from build123d import *

# Parameters (mm, degrees)
BOSS_EXTRUDE1_DEPTH = 5
CAVITY1_START       = -0.5
CAVITY1_OUTLINE_W   = 15
CAVITY1_OUTLINE_H   = 5
CAVITY1_DEPTH       = 5


# Read off the part's stored shape, not the designer's step: Cavity1
with BuildPart() as part:
    # Sketch1 → Boss-Extrude1 (new body)
    with BuildSketch(Plane.XY):
        Polygon((25, 1.5), (25, 4.5), (-25, 4.5), (-25, 1.5), (-20, 1.5), (-20, -1.5), (-25, -1.5), (-25, -4.5), (-6.424137908, -4.5), (-6.424137908, -9.5), (10.242528759, -9.5), (10.242528759, -4.5), (25, -4.5), (25, -1.5), (30, -1.5), (30, 1.5), align=None)
    extrude(amount=BOSS_EXTRUDE1_DEPTH)

    # Cavity1 outline → Cavity1 (cut)
    with BuildSketch(Plane(origin=(0, 0, 0), x_dir=(1, 0, 0), z_dir=(0, 1, 0)).offset(CAVITY1_START)):
        with Locations((2.5, -2.5)):
            Rectangle(CAVITY1_OUTLINE_W, CAVITY1_OUTLINE_H)
    extrude(amount=CAVITY1_DEPTH, mode=Mode.SUBTRACT)


solid = part.part
Here's how the part is built. I have some questions about the finished solid (model axes, mm). A direction names the side the tool comes from. Give positions to 0.01 mm unless a question says otherwise; leave off trailing zeros. Order: outer loops, then holes, each group sorted by start corner. A loop starts at its lowest first (then second) coordinate and runs counter-clockwise, first axis right, second up. Notation, with made-up numbers: (-1.75, 1) -> (14.25, 1) arc R16 cw to (14.25, 22) -> close; hole circle Ø4 at (80, -24). An arc over 180 degrees is marked (long way). One line per item, written item: value. Start each with the question number.
1. Imagine slicing it at D-D, the plane y = -4. List the corners of the cut face in (x, z) for me, plus the area to 3 significant figures.
2. Imagine slicing it at A-A, the plane y = 3.5. List the corners of the cut face in (x, z) for me, plus the area to 3 significant figures.
3. For faces 5 (the face through (25, 3, 2)), 6 (the face through (-16, -4.5, 2)), 7 (the face through (-23, 1.5, 2)), 8 (the face through (27, -1.5, 2)), which set-ups out of +Z, -Z, +X, -X, +Y, -Y let a thin tool reach every point of the face, with its end or its side?
4. Will these pins go through, and if not, where does the flat tip stop? pin 1 Ø1.5 at (y, z) = (-3.5, 2) entering from +X; pin 2 Ø6 at (x, y) = (-16, -5.5) entering from +Z; pin 3 Ø2 at (y, z) = (-8, 0.5) entering from -X; pin 4 Ø1.5 at (y, z) = (0, 1.5) entering from -X.
5. We'd pull the mould along X, two halves only. Please class faces 1 (the face through (10, 2, 3)), 2 (the face through (18, -4.5, 2)), 3 (the face through (-6.424, -7, 2)), 4 (the face through (-5, 2, 3)): released by +X, released by -X, zero draft, split by the parting line, or undercut.
6. Imagine slicing it at B-B, the plane z = 4.3. List the corners of the cut face in (x, y) for me.
7. I need wall thicknesses on probe 1 along X at (y, z) = (3.25, 4); probe 2 along X at (y, z) = (0.75, 1.5); probe 3 along Y at (x, z) = (-12.5, 4.1). Which ranges of each line are inside material? Lowest first, please. Write a range as from..to.
8. Imagine slicing it at C-C, the plane x = -3.5. List the corners of the cut face in (y, z) for me.
Values follow:
1. outline: (-25, 0) -> (25, 0) -> (25, 5) -> (-25, 5) -> close
1. area: 250 mm2
2. outline: (-25, 0) -> (-5, 0) -> (-5, 5) -> (-25, 5) -> close; (10, 0) -> (25, 0) -> (25, 5) -> (10, 5) -> close
2. area: 175 mm2
3. face 5: +Z, -Z, +X, +Y
3. face 6: +Z, -Z, -X, -Y
3. face 7: +Z, -Z, -X
3. face 8: +Z, -Z, +X, -Y
4. pin 1: stops at x = 25
4. pin 2: stops at z = 5
4. pin 3: stops at x = -6.42
4. pin 4: stops at x = -20
5. face 1: undercut
5. face 2: zero draft
5. face 3: released by -X
5. face 4: undercut
6. outline: (-25, -4.5) -> (-6.42, -4.5) -> (-6.42, -9.5) -> (10.24, -9.5) -> (10.24, -4.5) -> (25, -4.5) -> (25, -1.5) -> (30, -1.5) -> (30, 1.5) -> (25, 1.5) -> (25, 4.5) -> (10, 4.5) -> (10, -0.5) -> (-5, -0.5) -> (-5, 4.5) -> (-25, 4.5) -> (-25, 1.5) -> (-20, 1.5) -> (-20, -1.5) -> (-25, -1.5) -> close
7. probe 1: x = -25..-5, 10..25
7. probe 2: x = -20..-5, 10..30
7. probe 3: y = -4.5..4.5
8. outline: (-9.5, 0) -> (-0.5, 0) -> (-0.5, 5) -> (-9.5, 5) -> close
